from build123d import *

# Parameters (mm, degrees)
F0_R     = 22.225
F1_DEPTH = 25.4
F2_R     = 2.38125
F3_DEPTH = 6.35
F4_W     = 9.652
F4_H     = 9.652
F5_DEPTH = 12.7
F6_R     = 0.508
F7_SIZE  = 0.508


with BuildPart() as f1:
    # F0 (on Front) → F1 (new body)
    with BuildSketch(Plane.XZ):
        Circle(F0_R)
    extrude(amount=F1_DEPTH)

    # F2 (on face) → F3 (join)
    with BuildSketch(Plane.XZ.offset(25.4)):
        with Locations((0, 12.7)):
            Circle(F2_R)
        with Locations((-12.7, 0)):
            Circle(F2_R)
        with Locations((0, -12.7)):
            Circle(F2_R)
        with Locations((12.7, 0)):
            Circle(F2_R)
    extrude(amount=F3_DEPTH)

    # F4 (on face) → F5 (cut)
    with BuildSketch(Plane(origin=(0, 0, 0), x_dir=(-1, 0, 0), z_dir=(0, 1, 0))):
        Rectangle(F4_W, F4_H)
    extrude(amount=-F5_DEPTH, mode=Mode.SUBTRACT)

    # F6
    f6_edges = [f1.edges().sort_by_distance(p)[0] for p in [
        (-4.826, -6.35, -4.826),
        (-4.826, -6.35, 4.826),
        (4.826, -6.35, 4.826),
        (4.826, -6.35, -4.826),
    ]]
    fillet(f6_edges, radius=F6_R)

    # F7
    f7_edges = [f1.edges().sort_by_distance(p)[0] for p in [
        (0, 0, -4.826),
        (-22.225, 0, 0),
        (-22.225, -25.4, 0),
        (-15.08125, -31.75, 0),
        (-2.38125, -31.75, 12.7),
        (10.31875, -31.75, 0),
        (-2.38125, -31.75, -12.7),
    ]]
    chamfer(f7_edges, length=F7_SIZE)


solid = f1.part
For this review, take the finished solid that the model builds, in its own axes (mm). A direction names the side the tool comes from. Give positions to 0.01 mm unless a question says otherwise; leave off trailing zeros. Order: outer loops, then holes, each group sorted by start corner. A loop starts at its lowest first (then second) coordinate and runs counter-clockwise, first axis right, second up. Notation, with made-up numbers: (10.25, -27) - (61.25, -27) arc R20 cw to (61.25, -19) - close; hole circle Ø1 at (44.5, 34.5). An arc over 180 degrees is marked (long way). Answer as a JSON object with one key per item and string values. Group by question number.
Item 1: Machinability: for faces 4 (the flat face through (0, -25.4, 0)), 5 (the flat face through (-13, -31.75, 0)), 6 (the flat face through (4.826, -7, 0)), which of the approach directions +Z, -Z, +X, -X, +Y, -Y give a long, thin tool a straight path to every point of the face, cutting with its end or side? Answer none if there is none.
Item 2: Take a section at B-B on x = 0. Give the boundary of the cut face in (y, z) (3 decimals).
Item 3: Wall thickness on line 1 along Z through (x, y) = (0, -2.5) (3 decimals); line 2 along Y through (x, z) = (2.5, 14); line 3 along X through (y, z) = (-12.5, 3): over which ranges is each line inside the solid? List them lowest first.
Item 4: Take a section at C-C on y = -19.5. Give the boundary of the cut face in (x, z) (3 decimals), and give its area (3 significant figures).
Item 5: Clearance check with flat-ended pins moving along their axes: pin 1 Ø4 at (y, z) = (-24.5, -10) entering from +X; pin 2 Ø3 at (y, z) = (-22, 17.5) entering from -X; pin 3 Ø7 at (x, y) = (2, -3.5) entering from +Z (3 decimals). State where each tip first meets the part, or that it passes through.
Item 6: Draft analysis for pull direction Z (two halves, no side actions). For faces 1 (the flat face through (0, -12.7, 0)), 2 (the cylindrical face through (21.199, -12.529, 6.676)), 3 (the flat face through (0, -31.75, 13)), state which applies: pulls with the +Z half, pulls with the -Z half, needs draft (parallel to the pull), parting line crosses it, or undercut.
Item 7: Take a section at A-A on y = -11.5. Give the boundary of the cut face in (x, z) (3 decimals).
Reported:
{
 "1": {"face 4": "-Y", "face 5": "+Z, -Z, +X, -X, -Y", "face 6": "+Y"},
 "2": {"outline": "(-31.75, -14.573) - (-31.242, -15.081) - (-25.4, -15.081) - (-25.4, -21.717) - (-24.892, -22.225) - (-0.508, -22.225) - (0, -21.717) - (0, -5.334) - (-0.508, -4.826) - (-12.7, -4.826) - (-12.7, 4.826) - (-0.508, 4.826) - (0, 5.334) - (0, 21.717) - (-0.508, 22.225) - (-24.892, 22.225) - (-25.4, 21.717) - (-25.4, 15.081) - (-31.242, 15.081) - (-31.75, 14.573) - (-31.75, 10.827) - (-31.242, 10.319) - (-25.4, 10.319) - (-25.4, -10.319) - (-31.242, -10.319) - (-31.75, -10.827) - close"},
 "3": {"line 1": "-22.225 to -4.826, 4.826 to 22.225", "line 2": "-25.4 to 0", "line 3": "-22.02 to -4.83, 4.83 to 22.02"},
 "4": {"outline": "circle Ø44.45 at (0, 0)", "area": "1,550 mm^2"},
 "5": {"pin 1": "x = 20.74", "pin 2": "x = -15.43", "pin 3": "z = 22.225"},
 "6": {"face 1": "undercut", "face 2": "parting line crosses it", "face 3": "needs draft"},
 "7": {"outline": "circle Ø44.45 at (0, 0); hole (-4.826, -4.318) arc R0.508 ccw to (-4.318, -4.826) - (4.318, -4.826) arc R0.508 ccw to (4.826, -4.318) - (4.826, 4.318) arc R0.508 ccw to (4.318, 4.826) - (-4.318, 4.826) arc R0.508 ccw to (-4.826, 4.318) - close"}
}
